Build history of the part. All positions in model axes, mm. A direction names the side the tool comes from. Give positions to 0.01 mm unless a question says otherwise; leave off trailing zeros. Loops run counter-clockwise (first coordinate to the right, second up) from the corner with the lowest first, then second, coordinate; pieces in that order, holes last. Notation, with made-up numbers: (8.5, 71) - (29.5, 71) arc R24 ccw to (29.5, 94) - close; hole circle Ø11 at (81, 4). An arc over 180 degrees is marked (long way). Return JSON: item names as keys, results as strings. Group by question number.
1) Slice it at D-D (x = 28.5). List the corners of the cut face in (y, z), and give its area (3 significant figures).
2) Slice it at A-A (x = 13). List the corners of the cut face in (y, z), and give its area (3 significant figures).
3) Slice it at C-C (z = -29). List the corners of the cut face in (x, y), and give its area (3 significant figures).
4) 3-axis set-ups, long thin cutter, end or side, ignore diameter. For faces 4 (the face through (-5, 0, 0)), 5 (the face through (2.5, 10, -2.5)): which of +Z, -Z, +X, -X, +Y, -Y reach the whole face in a straight line?
5) Drop flat-ended pins along their axis: pin 1 (1.5 mm diameter, centred on x = 22.5, y = 16, fed in from -Z); pin 2 (20.5 mm diameter, centred on x = 8, z = -8, fed in from -Y); pin 3 (10 mm diameter, centred on y = 15, z = 8, fed in from -X); pin 4 (1.5 mm diameter, centred on x = 19.5, z = 19, fed in from -Y). Give the stop position or say it passes through.
6) Slice it at B-B (z = 10). List the corners of the cut face in (x, y).
7) Mould opens along X. For faces 1 (the face through (7.509, 4.93, 23.846)), 2 (the face through (2.42, 14.93, 1.55)), 3 (the face through (18, 10, -18)) say: released by +X, released by -X, zero draft, split by the parting line, or undercut.
8) Drill centre lines: probe 1 along X at (y, z) = (17.5, 0) (3 decimals); probe 2 along Y at (x, z) = (-20, 19); probe 3 along Z at (x, y) = (-1, 3.25). Where is each one in solid material? Low to high. Write a range as from..to.
```python
from build123d import *

# Parameters (mm, degrees)
SKETCH1_R           = 25
BOSS_EXTRUDE1_DEPTH = 10
SKETCH2_R           = 34
SKETCH2_R_2         = 2.875
BOSS_EXTRUDE2_DEPTH = 10


with BuildPart() as part:
    # Sketch1 → Boss-Extrude1 (new body)
    with BuildSketch(Plane(origin=(0, 0, 0), x_dir=(1, 0, 0), z_dir=(0, 1, 0))):
        with Locations(Location((0, 0, 0), (0, 0, 270))):
            Circle(SKETCH1_R)
        with BuildLine():
            Line((0, 4.5), (-0.922144385, 5.422144385))
            ThreePointArc((-0.922144385, 5.422144385), (-1.423504748, 5.312592045), (-1.912471729, 5.156786973))
            Line((-1.912471729, 5.156786973), (-2.25, 3.897114317))
            Line((-2.25, 3.897114317), (-3.509672656, 4.234642588))
            ThreePointArc((-3.509672656, 4.234642588), (-3.889087297, 3.889087297), (-4.234642588, 3.509672656))
            Line((-4.234642588, 3.509672656), (-3.897114317, 2.25))
            Line((-3.897114317, 2.25), (-5.156786973, 1.912471729))
            ThreePointArc((-5.156786973, 1.912471729), (-5.312592045, 1.423504748), (-5.422144385, 0.922144385))
            Line((-5.422144385, 0.922144385), (-4.5, 0))
            Line((-4.5, 0), (-5.422144385, -0.922144385))
            ThreePointArc((-5.422144385, -0.922144385), (-5.312592045, -1.423504748), (-5.156786973, -1.912471729))
            Line((-5.156786973, -1.912471729), (-3.897114317, -2.25))
            Line((-3.897114317, -2.25), (-4.234642588, -3.509672656))
            ThreePointArc((-4.234642588, -3.509672656), (-3.889087297, -3.889087297), (-3.509672656, -4.234642588))
            Line((-3.509672656, -4.234642588), (-2.25, -3.897114317))
            Line((-2.25, -3.897114317), (-1.912471729, -5.156786973))
            ThreePointArc((-1.912471729, -5.156786973), (-1.423504748, -5.312592045), (-0.922144385, -5.422144385))
            Line((-0.922144385, -5.422144385), (0, -4.5))
            Line((0, -4.5), (0.922144385, -5.422144385))
            ThreePointArc((0.922144385, -5.422144385), (1.423504748, -5.312592045), (1.912471729, -5.156786973))
            Line((1.912471729, -5.156786973), (2.25, -3.897114317))
            Line((2.25, -3.897114317), (3.509672656, -4.234642588))
            ThreePointArc((3.509672656, -4.234642588), (3.889087297, -3.889087297), (4.234642588, -3.509672656))
            Line((4.234642588, -3.509672656), (3.897114317, -2.25))
            Line((3.897114317, -2.25), (5.156786973, -1.912471729))
            ThreePointArc((5.156786973, -1.912471729), (5.312592045, -1.423504748), (5.422144385, -0.922144385))
            Line((5.422144385, -0.922144385), (4.5, 0))
            Line((4.5, 0), (5.422144385, 0.922144385))
            ThreePointArc((5.422144385, 0.922144385), (5.312592045, 1.423504748), (5.156786973, 1.912471729))
            Line((5.156786973, 1.912471729), (3.897114317, 2.25))
            Line((3.897114317, 2.25), (4.234642588, 3.509672656))
            ThreePointArc((4.234642588, 3.509672656), (3.889087297, 3.889087297), (3.509672656, 4.234642588))
            Line((3.509672656, 4.234642588), (2.25, 3.897114317))
            Line((2.25, 3.897114317), (1.912471729, 5.156786973))
            ThreePointArc((1.912471729, 5.156786973), (1.423504748, 5.312592045), (0.922144385, 5.422144385))
            Line((0.922144385, 5.422144385), (0, 4.5))
        make_face(mode=Mode.SUBTRACT)
    extrude(amount=BOSS_EXTRUDE1_DEPTH)

    # Sketch2 → Boss-Extrude2 (add)
    with BuildSketch(Plane(origin=(0, 10, 0), x_dir=(1, 0, 0), z_dir=(0, 1, 0))):
        with Locations(Location((0, 0, 0), (0, 0, 270))):
            Circle(SKETCH2_R)
        with Locations(Location((0, 0, 0), (0, 0, 270))):
            Circle(SKETCH2_R_2, mode=Mode.SUBTRACT)
    extrude(amount=BOSS_EXTRUDE2_DEPTH)


solid = part.part
```
Results:
{
 "1": {"outline": "(10, -18.54) - (20, -18.54) - (20, 18.54) - (10, 18.54) - close", "area": "371 mm2"},
 "2": {"outline": "(0, -21.35) - (10, -21.35) - (10, -31.42) - (20, -31.42) - (20, 31.42) - (10, 31.42) - (10, 21.35) - (0, 21.35) - close", "area": "1,060 mm2"},
 "3": {"outline": "(-17.75, 10) - (17.75, 10) - (17.75, 20) - (-17.75, 20) - close", "area": "355 mm2"},
 "4": {"face 4": "+Z, -Z, +X, -X, -Y", "face 5": "-Y"},
 "5": {"pin 1": "z = -26.13", "pin 2": "y = 0", "pin 3": "x = -33.87", "pin 4": "y = 10"},
 "6": {"outline": "(-32.5, 10) - (-22.91, 10) - (-22.91, 0) - (22.91, 0) - (22.91, 10) - (32.5, 10) - (32.5, 20) - (-32.5, 20) - close"},
 "7": {"face 1": "split by the parting line", "face 2": "undercut", "face 3": "zero draft"},
 "8": {"probe 1": "-34..-2.875, 2.875..34", "probe 2": "10..20", "probe 3": "-24.98..-5.41, 5.41..24.98"}
}
